The listing builds one solid part. Answer for the finished solid, in the listing's coordinates (mm). A direction names the side the tool comes from. Coordinates: 2 decimals unless noted, no trailing zeros. Write each loop counter-clockwise with the first axis right and the second up, starting at its lowest first coordinate (ties: lowest second). Pieces come first, ordered by that corner, then holes.
Autodesk Inventor part; units mm, degrees
ref_plane "Arbeitsebene1" through (0, 6, 0) normal (0, 1, 0) x (-1, 0, 0)
ref_plane "YZ Plane" through (0, 0, 0) normal (1, 0, 0) x (0, 1, 0)
ref_plane "XY Plane" through (0, 0, 0) normal (0, 0, 1) x (1, 0, 0)
sketch "Skizze1" plane through (0, 0, 0) normal (0, 0, 1) x (1, 0, 0)
  line L0 (-9.8448, 0) -> (9.4061, 0)
  line L1 (-2.4, 4.025) -> (2.4, 4.025)
  line L2 (2.5, 4.125) -> (2.5, 5.9)
  line L3 (2.4, 6) -> (-2.4, 6)
  line L4 (-2.5, 5.9) -> (-2.5, 4.125)
  line L5 (0, 0) -> (0, 4.025) construction
  line L6 (-2.4, 4.025) -> (-2.5, 4.125)
  line L7 (2.4, 4.025) -> (2.5, 4.125)
  line L8 (2.5, 5.9) -> (2.4, 6)
  line L9 (-2.4, 6) -> (-2.5, 5.9)
  point P0 (-2.5, 4.025)
  point P1 (2.5, 6)
  point P2 (2.5, 4.025)
  point P3 (-2.5, 6)
  dimension "d0" = 0.1
  dimension "d1" = 0.1
  dimension "d2" = 0.1
  dimension "d3" = 0.1
  dimension "d4" = 0.1
  dimension "d5" = 0.1
  dimension "d6" = 0.1
  dimension "d7" = 0.1
  dimension "d8" = 8.05
  dimension "d9" = 12
  dimension "d10" = 5
revolve "Umdrehung1" add sketch "Skizze1" angle 360 about axis through (-9.8448, 0, 0) along (1, 0, 0)
ref_plane "Arbeitsebene1" through (0, 6, 0) normal (0, 1, 0) x (-1, 0, 0)
sketch "Skizze2" plane through (0, 6, 0) normal (0, 1, 0) x (-1, 0, 0)
  point P0 (0, 0)
  point P1 (0, 0)
hole "Bohrung1" at (0, 6, 0) direction (0, -1, 0) diameter 2.459 end up to surface
properties part number "pos-ring_d8_D12_t5_M3_V1" material "Messing, weicher Gelbton"
(1) Each of these flat-tipped pins is pushed along its axis until it touches: pin 1 (1.5 mm diameter, centred on x = 0, z = 0, fed in from +Y); pin 2 (2 mm diameter, centred on x = -1.5, z = -4.5, fed in from -Y); pin 3 (1.5 mm diameter, centred on x = -1.5, y = -3.5, fed in from +Z). Where does it stop, or does it pass through?
(2) Section D-D, the plane x = -0.7 is taken. Write down the section's boundary in (y, z) (3 decimals), plus the area to 3 significant figures.
(3) Find the intervals of material crossed by probe 1 along Z at (x, y) = (0.4, 0) (3 decimals); probe 2 along X at (y, z) = (4.45, 0); probe 3 along Z at (x, y) = (0, 5.35), in increasing order.
(4) Section A-A, the plane z = 0 is taken. State how many separate pieces and enclosed holes the cut face has, plus the area to 3 significant figures.
(5) Section B-B, the plane y = 0 is taken. Write down the section's boundary in (x, z) (3 decimals).
(6) Section C-C, the plane x = -1.7 is taken. Write down the section's boundary in (y, z) (3 decimals).
(7) Which of the six approach directions +Z, -Z, +X, -X, +Y, -Y give full straight-line access (tool end or side, diameter ignored) to faces 1 (the flat face through (2.5, 3, -4)), 2 (the cylindrical face through (-0.05, 4.9, -1.23))?
(8) For a pull along Z with two mould halves and no side action, classify faces 3 (the cylindrical face through (0, -6, 0)), 4 (the cylindrical face through (0.03, -4.02, 0.18)), 5 (the flat face through (-2.5, 3, -4)) as pulls with the +Z half, pulls with the -Z half, needs draft (parallel to the pull), parting line crosses it, or undercut.
Solution:
1. pin 1: stops at y = -3.95
1. pin 2: stops at y = -4.87
1. pin 3: stops at z = 5.33
2. outline: (3.896, -1.011) arc R4.025 cw (long way) to (3.896, 1.011) - (5.914, 1.011) arc R6 ccw (long way) to (5.914, -1.011) - close
2. area: 58.2 mm2
3. probe 1: z = -6 to -4.025, 4.025 to 6
3. probe 2: x = -2.5 to -1.23, 1.23 to 2.5
3. probe 3: z = -2.72 to -1.23, 1.23 to 2.72
4. separate pieces: 3
4. enclosed holes: 0
4. area: 14.9 mm2
5. outline: (-2.5, -5.9) - (-2.4, -6) - (2.4, -6) - (2.5, -5.9) - (2.5, -4.125) - (2.4, -4.025) - (-2.4, -4.025) - (-2.5, -4.125) - close; (-2.5, 4.125) - (-2.4, 4.025) - (2.4, 4.025) - (2.5, 4.125) - (2.5, 5.9) - (2.4, 6) - (-2.4, 6) - (-2.5, 5.9) - close
6. outline: circle Ø12 at (0, 0); hole circle Ø8.05 at (0, 0)
7. face 1: +Z, -Z, +X, +Y, -Y
7. face 2: +Y
8. face 3: parting line crosses it
8. face 4: undercut
8. face 5: needs draft
